Autodesk Inventor part; units mm, degrees
ref_plane "YZ Plane" through (0, 0, 0) normal (1, 0, 0) x (0, 1, 0)
ref_plane "XZ Plane" through (0, 0, 0) normal (0, 1, 0) x (-1, 0, 0)
ref_plane "XY Plane" through (0, 0, 0) normal (0, 0, 1) x (1, 0, 0)
sketch "Sketch1" plane through (0, 0, 0) normal (0, 1, 0) x (-1, 0, 0)
  line L0 (64.2199, -131.5556) -> (64.2199, -221.5556)
  line L1 (3.3449, -196.5556) -> (3.3449, -176.5556)
  circle A0 centre (9.8449, -186.5556) radius 1.5
  line L2 (-9.1551, -221.5556) -> (-9.1551, -201.5556)
  circle A1 centre (21.8449, -186.5556) radius 1.5
  line L3 (3.3449, -176.5556) -> (28.3449, -176.5556)
  line L4 (28.3449, -196.5556) -> (3.3449, -196.5556)
  line L5 (28.3449, -176.5556) -> (28.3449, -196.5556)
  line L6 (64.2199, -221.5556) -> (-55.7801, -221.5556)
  line L7 (-9.1551, -201.5556) -> (40.8449, -201.5556)
  line L8 (40.8449, -221.5556) -> (-9.1551, -221.5556)
  circle A2 centre (58.2199, -214.0556) radius 1.5
  line L9 (40.8449, -201.5556) -> (40.8449, -221.5556)
  line L10 (30.8449, -173.5556) -> (15.8449, -173.5556)
  line L11 (15.8449, -173.5556) -> (15.8449, -143.5556)
  line L12 (15.8449, -143.5556) -> (30.8449, -143.5556)
  line L13 (30.8449, -143.5556) -> (30.8449, -173.5556)
  line L14 (0.8449, -173.5556) -> (15.8449, -173.5556)
  circle A3 centre (8.3449, -164.5556) radius 1.5
  circle A4 centre (8.3449, -152.5556) radius 1.5
  circle A5 centre (23.3449, -164.5556) radius 1.5
  line L15 (0.8449, -143.5556) -> (0.8449, -173.5556)
  line L16 (15.8449, -173.5556) -> (15.8449, -143.5556)
  line L17 (15.8449, -143.5556) -> (0.8449, -143.5556)
  circle A6 centre (23.3449, -152.5556) radius 1.5
  line L18 (49.2199, -166.2056) -> (64.2199, -166.2056)
  circle A7 centre (53.7199, -158.7056) radius 1.5
  circle A8 centre (53.7199, -158.7056) radius 2.5
  circle A9 centre (59.7199, -158.7056) radius 1.5
  circle A10 centre (59.7199, -158.7056) radius 2.5
  line L19 (49.2199, -151.2056) -> (49.2199, -166.2056)
  line L20 (64.2199, -166.2056) -> (64.2199, -151.2056)
  line L21 (64.2199, -151.2056) -> (49.2199, -151.2056)
  line L22 (64.2199, -148.5556) -> (64.2199, -131.5556)
  line L23 (64.2199, -131.5556) -> (49.2199, -131.5556)
  line L24 (-55.7801, -221.5556) -> (-55.7801, -131.5556)
  line L25 (-55.7801, -131.5556) -> (-6.8176, -131.5556)
  line L26 (-55.7801, -176.5556) -> (-55.7801, -171.5556)
  line L27 (-55.7801, -171.5556) -> (-55.7801, -181.5556)
  circle A11 centre (-49.7801, -215.5556) radius 1.5
  circle A12 centre (-49.7801, -155.6806) radius 1.5
  circle A13 centre (-49.7801, -155.6806) radius 2.5
  line L28 (-41.5051, -176.5556) -> (-60.5551, -176.5556) construction
  circle A14 centre (-49.7801, -197.4306) radius 2.5
  circle A15 centre (-49.7801, -197.4306) radius 1.5
  line L29 (3.1824, -131.5556) -> (64.2199, -131.5556)
  circle A16 centre (36.7199, -137.5556) radius 2.5
  circle A17 centre (36.7199, -137.5556) radius 1.5
  line L30 (3.1824, -131.5556) -> (-6.8176, -131.5556)
  circle A18 centre (-5.0301, -137.5556) radius 1.5
  circle A19 centre (-5.0301, -137.5556) radius 2.5
  line L31 (15.8449, -176.5556) -> (15.8449, -139.0556) construction
  line L32 (49.2199, -151.2056) -> (41.2199, -151.2056)
  line L33 (41.2199, -151.2056) -> (41.2199, -131.5556)
  point P0 (0, -174.625)
  point P1 (-1.8176, -176.5556)
  point P2 (3.3449, -186.5556)
  point P3 (36.7199, -143.5556)
  point P4 (-5.0301, -143.5556)
  point P5 (-9.1551, -221.5556)
  point P6 (44.2199, -131.5556)
  dimension "d32" = 12
  dimension "d33" = 7.5
  dimension "d34" = 7.5
  dimension "d35" = 12
  dimension "d36" = 0
  dimension "d37" = 0
  dimension "d39" = 8
extrude "Extrusion1" add sketch "Sketch1" along normal blind 4 contours L33 L32 L19 L18 L0 L6 L9 L7 L2 L24 L25 L30 L29 | L1 L3 L5 L4 | A0 | A1 | L10 L11 L12 L13 | L14 L15 L17 L11 | A3 | A4 | A5 | A6
extrude "Extrusion2" add sketch "Sketch1" along normal blind 2 contours L0 L18 L19 L21 | L1 L3 L5 L4 | L10 L11 L12 L13 | L14 L15 L17 L11 | A8 | A10 | A13 | A14 | A16 | A19
properties part number "Casis Kanan Atas_3DPrint"
Geometry check sheet. Reference: the model listing, model coordinates, mm. A direction names the side the tool comes from. Coordinates: 2 decimals unless noted, no trailing zeros. Order: outer loops, then holes, each group sorted by start corner. A loop starts at its lowest first (then second) coordinate and runs counter-clockwise, first axis right, second up. Notation, with made-up numbers: M 11,17.5 L 35,17.5 A19 cw 35,28.5 Z; hole C 83,-33 d10. An arc over 180 degrees is marked long. Use CSV: the item, a comma, the result in double quotes.
Item 1: Thickness scan on line 1 along X through (y, z) = (2.35, -214); line 2 along X through (y, z) = (3.3, -215); line 3 along X through (y, z) = (2.65, -216). Record the ranges inside material, lowest first.
Returned:
line 1,"x = -64.22 to -59.72, -56.72 to -40.84, 9.16 to 55.78"
line 2,"x = -64.22 to -59.39, -57.05 to -40.84, 9.16 to 48.39, 51.17 to 55.78"
line 3,"x = -64.22 to -40.84, 9.16 to 48.35, 51.21 to 55.78"
Item 2: Cross-section at A-A on y = 3.4. Record the cut outline in (x, z), then the cut area to 3 significant figures.
Returned:
outline,"M -64.22,-221.56 L -40.84,-221.56 L -40.84,-201.56 L 9.16,-201.56 L 9.16,-221.56 L 55.78,-221.56 L 55.78,-131.56 L -41.22,-131.56 L -41.22,-151.21 L -49.22,-151.21 L -49.22,-166.21 L -64.22,-166.21 Z; hole C -58.22,-214.06 d3; hole C -36.72,-137.56 d5; hole C 5.03,-137.56 d5; hole C 49.78,-197.43 d5; hole C 49.78,-155.68 d5; hole C 49.78,-215.56 d3"
area,"9,030 mm2"
Item 3: Gauge pin test, flat ends, axial feed: pin 1 Ø2.5 at (x, z) = (6, -137) entering from +Y; pin 2 Ø4 at (x, z) = (-37.5, -138.5) entering from +Y; pin 3 Ø1 at (x, y) = (-58.5, 3) entering from +Z; pin 4 Ø2 at (x, y) = (-47.5, 2.5) entering from +Z. Record the tip position at first contact, or that the pin passes through.
Returned:
pin 1,"stops at y = 2"
pin 2,"stops at y = 4"
pin 3,"stops at z = -166.21"
pin 4,"stops at z = -151.21"
Item 4: Cross-section at C-C on x = -24.5. Record the cut outline in (y, z).
Returned:
outline,"M 0,-201.56 L 4,-201.56 L 4,-131.56 L 0,-131.56 Z"
Item 5: Cross-section at B-B on z = -148. Record the cut outline in (x, y), then the cut area to 3 significant figures.
Returned:
outline,"M -41.22,0 L 55.78,0 L 55.78,4 L -41.22,4 Z"
area,"388 mm2"
Item 6: Mould release check, pull along Z, two halves, no side actions. Record for faces 1 (the flat face through (9.155, 2, -212)), 2 (the cylindrical face through (-36.395, 0.986, -136.091)), 3 (the flat face through (-15, 2, -201.556)): pulls with the +Z half, pulls with the -Z half, needs draft (parallel to the pull), parting line crosses it, or undercut.
Returned:
face 1,"needs draft"
face 2,"undercut"
face 3,"pulls with the -Z half"
Item 7: Tool access check on faces 4 (the flat face through (-41.22, 2, -142)), 5 (the cylindrical face through (-54.412, 0.986, -157.375)), 6 (the flat face through (-38, 2, -139)). Record the directions out of +Z, -Z, +X, -X, +Y, -Y that give a thin tool (end or side, any length) a straight path to the whole face; none if there is none.
Returned:
face 4,"+Z, -X, +Y, -Y"
face 5,"+Y, -Y"
face 6,"+Y"
